Here's how the part is built. I have some questions about the finished solid (model axes, mm). Face numbers are marked on the shaded views. A direction names the side the tool comes from. Give positions to 0.01 mm unless a question says otherwise; leave off trailing zeros. Write each loop counter-clockwise with the first axis right and the second up, starting at its lowest first coordinate (ties: lowest second). Pieces come first, ordered by that corner, then holes. Notation, with made-up numbers: (-12.5, 62.5) - (-4.5, 62.5) arc R31 cw to (-4.5, 87.5) - close; hole circle Ø11 at (-23, 50). An arc over 180 degrees is marked (long way). Use one line per item in the form item = value. Start each with the question number.
from build123d import *

# Parameters (mm, degrees)
F0_W        = 88.9
F0_H        = 12.446
F1_DEPTH    = 2.54
F2_W        = 5.08
F2_H        = 12.446
F3_DEPTH    = 7.62
F4_T1_DEPTH = 37.846
F4_T3_DEPTH = 7.62


# Not quite as in the source:
# - a fillet or chamfer that OpenCascade refuses, or shapes differently, is made with other operations: its cross-section is extruded or revolved along the edge and cut away or added


with BuildPart() as f1:
    # F0 (on Top) → F1 (new body)
    with BuildSketch(Plane.XY):
        with Locations((-4.0042309799, -31.983400695)):
            Rectangle(F0_W, F0_H)
    extrude(amount=F1_DEPTH)

    # F2 (on face) → F3 (join)
    with BuildSketch(Plane.XY.offset(2.54)):
        with Locations((-45.9142309799, -31.983400695)):
            Rectangle(F2_W, F2_H)
        with Locations((-33.2142309799, -31.983400695)):
            Rectangle(F2_W, F2_H)
        with Locations((-20.5142309799, -31.983400695)):
            Rectangle(F2_W, F2_H)
        with Locations((-7.8142309799, -31.983400695)):
            Rectangle(F2_W, F2_H)
        with Locations((4.8857690201, -31.983400695)):
            Rectangle(F2_W, F2_H)
        with Locations((17.5857690201, -31.983400695)):
            Rectangle(F2_W, F2_H)
    extrude(amount=F3_DEPTH)

    # F4: fillet of radius 5.08 on 7 edges, made by hand

    # F4_s2 → F4_t1 (cut)
    with BuildSketch(Plane.XZ.offset(13.060400695)):
        with BuildLine():
            ThreePointArc((-48.4542309799, 5.08), (-46.9663334283, 8.6721024484), (-43.3742309799, 10.16))
            Line((-43.3742309799, 10.16), (-48.4542309799, 10.16))
            Line((-48.4542309799, 10.16), (-48.4542309799, 5.08))
        make_face()
        with BuildLine():
            ThreePointArc((-30.6742309799, 10.16), (-34.2663334283, 8.6721024484), (-35.7542309799, 5.08))
            Line((-35.7542309799, 5.08), (-35.7542309799, 10.16))
            Line((-35.7542309799, 10.16), (-30.6742309799, 10.16))
        make_face()
        with BuildLine():
            ThreePointArc((-17.9742309799, 10.16), (-21.5663334283, 8.6721024484), (-23.0542309799, 5.08))
            Line((-23.0542309799, 5.08), (-23.0542309799, 10.16))
            Line((-23.0542309799, 10.16), (-17.9742309799, 10.16))
        make_face()
        with BuildLine():
            ThreePointArc((-5.2742309799, 10.16), (-8.8663334283, 8.6721024484), (-10.3542309799, 5.08))
            Line((-10.3542309799, 5.08), (-10.3542309799, 10.16))
            Line((-10.3542309799, 10.16), (-5.2742309799, 10.16))
        make_face()
        with BuildLine():
            ThreePointArc((7.4257690201, 10.16), (3.8336665717, 8.6721024484), (2.3457690201, 5.08))
            Line((2.3457690201, 5.08), (2.3457690201, 10.16))
            Line((2.3457690201, 10.16), (7.4257690201, 10.16))
        make_face()
        with BuildLine():
            ThreePointArc((20.1257690201, 10.16), (16.5336665717, 8.6721024484), (15.0457690201, 5.08))
            Line((15.0457690201, 5.08), (15.0457690201, 10.16))
            Line((15.0457690201, 10.16), (20.1257690201, 10.16))
        make_face()
    extrude(amount=F4_T1_DEPTH, mode=Mode.SUBTRACT)

    # F4_s4 → F4_t3 (cut)
    with BuildSketch(Plane.YZ.offset(-30.6742309799)):
        with BuildLine():
            ThreePointArc((-30.840400695, 2.54), (-27.2482982466, 1.0521024484), (-25.760400695, -2.54))
            Line((-25.760400695, -2.54), (-25.760400695, 2.54))
            Line((-25.760400695, 2.54), (-30.840400695, 2.54))
        make_face()
    extrude(amount=F4_T3_DEPTH, mode=Mode.SUBTRACT)


solid = f1.part
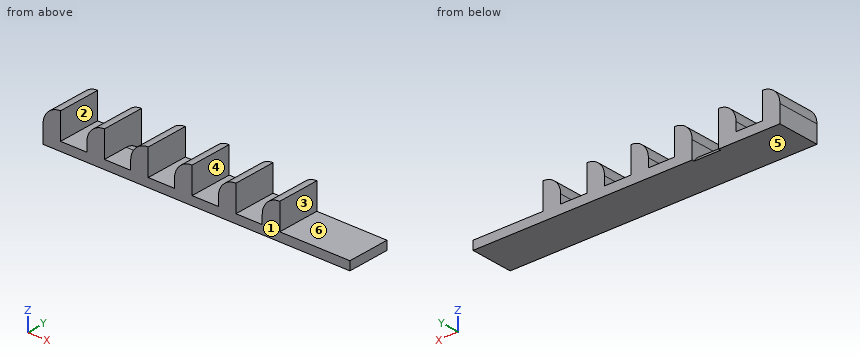
1. I want a section at B-B, the plane y = -28. List the corners of the cut face in (x, z) for me.
2. We'd pull the mould along X, two halves only. Please class the marked faces 1, 2 and 3: pulls with the +X half, pulls with the -X half, needs draft (parallel to the pull), parting line crosses it, or undercut.
3. I want a section at C-C, the plane x = -26. List the corners of the cut face in (y, z) for me.
4. For the marked faces 4, 5 and 6, which set-ups out of +Z, -Z, +X, -X, +Y, -Y let a thin tool reach every point of the face, with its end or its side?
5. I want a section at D-D, the plane y = -33.5. List the corners of the cut face in (x, z) for me.
6. I want a section at A-A, the plane z = 7.25. List the corners of the cut face in (x, y) for me.
7. For P1, Ø3.5, axis at x = 27, y = -31.5, coming from the +Z side; P2, Ø2, axis at y = -34.5, z = 8, coming from the +X side; P3, Ø6, axis at x = -25.5, y = -34.5, coming from the +Z side, each with a flat end and sliding along its axis, tell me the tip position at first contact or that it passes through.
8. Please list where these lines run through material, in increasing order: line 1 (X direction, y = -27, z = 5); line 2 (X direction, y = -28.25, z = 2.5); line 3 (Z direction, x = -39.5, y = -29.75).
Result sheet:
q1.outline = (-48.45, 0) - (40.45, 0) - (40.45, 2.54) - (20.13, 2.54) - (20.13, 10.16) arc R5.08 ccw to (15.05, 5.08) - (15.05, 2.54) - (7.43, 2.54) - (7.43, 10.16) arc R5.08 ccw to (2.35, 5.08) - (2.35, 2.54) - (-5.27, 2.54) - (-5.27, 10.16) arc R5.08 ccw to (-10.35, 5.08) - (-10.35, 2.54) - (-17.97, 2.54) - (-17.97, 10.16) arc R5.08 ccw to (-23.05, 5.08) - (-23.05, 1.67) - (-30.67, 1.67) - (-30.67, 10.16) arc R5.08 ccw to (-35.75, 5.08) - (-35.75, 2.54) - (-43.37, 2.54) - (-43.37, 10.16) arc R5.08 ccw to (-48.45, 5.08) - close
q2.face_1 = needs draft
q2.face_2 = undercut
q2.face_3 = pulls with the +X half
q3.outline = (-38.21, 0) - (-26.44, 0) arc R5.08 ccw to (-30.84, 2.54) - (-38.21, 2.54) - close
q4.face_4 = +Z, +Y, -Y
q4.face_5 = -Z, +X, -X, +Y, -Y
q4.face_6 = +Z, +X, +Y, -Y
q5.outline = (-48.45, 0) - (40.45, 0) - (40.45, 2.54) - (20.13, 2.54) - (20.13, 10.16) arc R5.08 ccw to (15.05, 5.08) - (15.05, 2.54) - (7.43, 2.54) - (7.43, 10.16) arc R5.08 ccw to (2.35, 5.08) - (2.35, 2.54) - (-5.27, 2.54) - (-5.27, 10.16) arc R5.08 ccw to (-10.35, 5.08) - (-10.35, 2.54) - (-17.97, 2.54) - (-17.97, 10.16) arc R5.08 ccw to (-23.05, 5.08) - (-23.05, 2.54) - (-30.67, 2.54) - (-30.67, 10.16) arc R5.08 ccw to (-35.75, 5.08) - (-35.75, 2.54) - (-43.37, 2.54) - (-43.37, 10.16) arc R5.08 ccw to (-48.45, 5.08) - close
q6.outline = (-47.97, -38.21) - (-43.37, -38.21) - (-43.37, -25.76) - (-47.97, -25.76) - close; (-35.27, -38.21) - (-30.67, -38.21) - (-30.67, -25.76) - (-35.27, -25.76) - close; (-22.57, -38.21) - (-17.97, -38.21) - (-17.97, -25.76) - (-22.57, -25.76) - close; (-9.87, -38.21) - (-5.27, -38.21) - (-5.27, -25.76) - (-9.87, -25.76) - close; (2.83, -38.21) - (7.43, -38.21) - (7.43, -25.76) - (2.83, -25.76) - close; (15.53, -38.21) - (20.13, -38.21) - (20.13, -25.76) - (15.53, -25.76) - close
q7.P1 = 2.54
q7.P2 = 20.13
q7.P3 = 7.39
q8.line_1 = -48.45 to -43.37, -35.75 to -30.67, -23.05 to -17.97, -10.35 to -5.27, 2.35 to 7.43, 15.05 to 20.13
q8.line_2 = -48.45 to -30.67, -23.05 to 40.45
q8.line_3 = 0 to 2.54
